```python
from build123d import *

# Parameters (mm, degrees)
F0_W     = 19.05
F0_H     = 1847.85
F1_DEPTH = 374.65
F3_DEPTH = 374.651


with BuildPart() as f1:
    # F0 (on Front) → F1 (new body)
    with BuildSketch(Plane.XZ):
        with Locations((-9.525, 923.925)):
            Rectangle(F0_W, F0_H)
    extrude(amount=F1_DEPTH)

    # F2 (on face) → F3 (cut, through all)
    with BuildSketch(Plane(origin=(0, 0, 0), x_dir=(-1, 0, 0), z_dir=(0, 1, 0))):
        with BuildLine():
            ThreePointArc((6.35, 103.1133947655), (4.7389469003, 156.5427900913), (0, 209.7859883352))
            Line((0, 209.7859883352), (0, 82.55))
            Line((0, 82.55), (6.35, 82.55))
            Line((6.35, 82.55), (6.35, 101.6))
            Line((6.35, 101.6), (6.35, 103.1133947655))
        make_face()
        Polygon((0, 82.55), (0, 209.7859883352), (-25.7673989981, 209.7859883352), (-37.0378904045, 82.55), align=None)
    extrude(amount=-F3_DEPTH, mode=Mode.SUBTRACT)


solid = f1.part
```
Geometry check sheet. Reference: the model listing, model coordinates, mm. A direction names the side the tool comes from. Give positions to 0.01 mm unless a question says otherwise; leave off trailing zeros. Write each loop counter-clockwise with the first axis right and the second up, starting at its lowest first coordinate (ties: lowest second). Pieces come first, ordered by that corner, then holes. Notation, with made-up numbers: (-14.5, 6.5) -> (3.5, 6.5) arc R6 ccw to (3.5, 17.5) -> close; hole circle Ø9 at (71.5, -25). An arc over 180 degrees is marked (long way). Use one line per item in the form item = value.
Item 1: Scan lines: line 1 (X direction, y = -327, z = 186); line 2 (X direction, y = -331, z = 192). Record each from-to range of solid material in increasing order.
Results list:
line_1 = -19.05 to -2.51
line_2 = -19.05 to -1.93
Item 2: Sectioned sample at A-A on y = -150. Enter the section's corners in (x, z).
Results list:
outline = (-19.05, 0) -> (0, 0) -> (0, 82.55) -> (-6.35, 82.55) -> (-6.35, 103.11) arc R911.87 cw to (0, 209.79) -> (0, 1847.85) -> (-19.05, 1847.85) -> close
Item 3: Access from +Z, -Z, +X, -X, +Y, -Y to the whole of each face (thin tool, end or side, straight path). Record for faces 1 (the cylindrical face through (-4.783, -184.702, 155.796)), 2 (the flat face through (-19.05, -185, 911)).
Results list:
face_1 = +X, +Y, -Y
face_2 = +Z, -Z, -X, +Y, -Y
Item 4: Depth check by flat-ended pin: pin 1 Ø10.5 at (y, z) = (-166.5, 90.5) entering from +X. Enter the tip coordinate at first touch or a pass-through.
Results list:
pin_1 = -6.35
